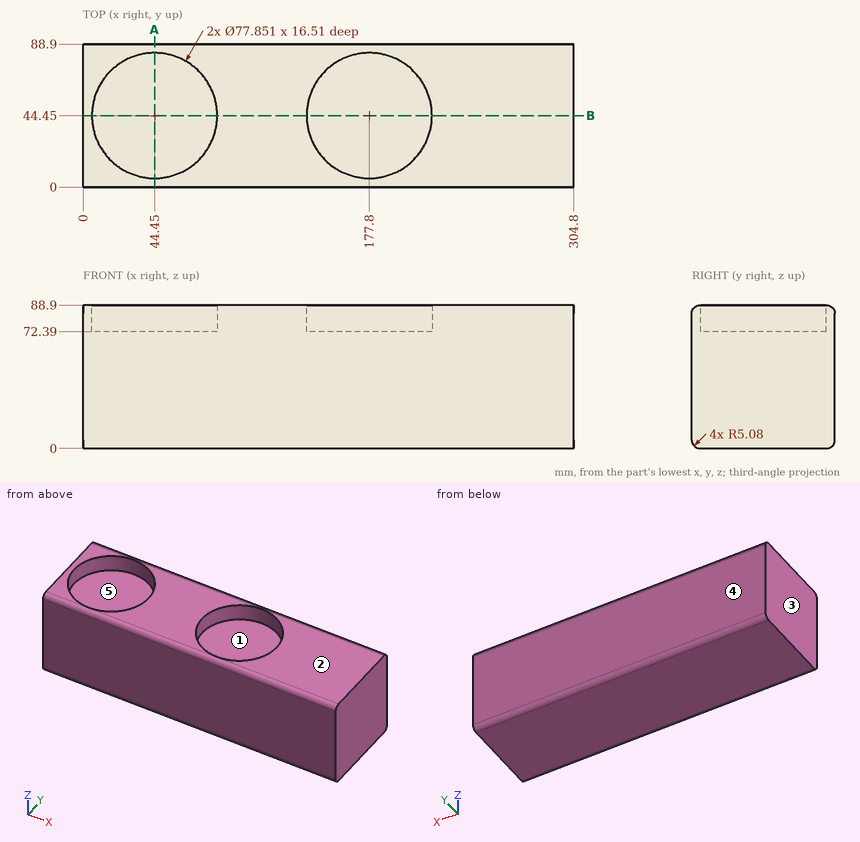
Here's the drawing with two shaded views (mm, measured from the low corner). I have some questions. A direction names the side the tool comes from. Round coordinates to 2 decimals unless told otherwise and drop trailing zeros. Write each loop counter-clockwise with the first axis right and the second up, starting at its lowest first coordinate (ties: lowest second). Pieces come first, ordered by that corner, then holes. Notation, with made-up numbers: M -18,14 L -12,14 A20 cw -12,22 Z; hole C -20,34.5 d9. An arc over 180 degrees is marked long. Use CSV: the item, a comma, the result in double quotes.
(1) I'm going to push flat-ended pins straight in: pin 1 (8 mm diameter, centred on x = 180, z = 49.5, fed in from -Y); pin 2 (1.5 mm diameter, centred on x = 210, y = 33, fed in from +Z). Where does each tip first touch, or does it pass through?
Check values:
pin 1,"y = 0"
pin 2,"z = 72.39"
(2) Imagine slicing it at A-A (x = 44.45). Write out the boundary of the cut face in (y, z).
Check values:
outline,"M 0,5.08 A5.08 ccw 5.08,0 L 83.82,0 A5.08 ccw 88.9,5.08 L 88.9,83.82 A5.08 ccw 83.82,88.9 L 83.38,88.9 L 83.38,72.39 L 5.52,72.39 L 5.52,88.9 L 5.08,88.9 A5.08 ccw 0,83.82 Z"
(3) We'd pull the mould along X, two halves only. Please class the marked faces 1, 2 and 3: +X half, -X half, draft (parallel to the pull), parting line (faces both ways), or undercut.
Check values:
face 1,"undercut"
face 2,"draft"
face 3,"-X half"
(4) I need wall thicknesses on line 1 along Y through (x, z) = (44.45, 77); line 2 along Z through (x, y) = (62, 77.5); line 3 along Y through (x, z) = (182, 72.5). Which ranges of each line are inside material? Lowest first, please.
Check values:
line 1,"0 to 5.52, 83.38 to 88.9"
line 2,"0 to 72.39"
line 3,"0 to 5.75, 83.15 to 88.9"
(5) Imagine slicing it at B-B (y = 44.45). Write out the boundary of the cut face in (x, z), plus the area to 3 significant figures.
Check values:
outline,"M 0,0 L 304.8,0 L 304.8,88.9 L 216.73,88.9 L 216.73,72.39 L 138.87,72.39 L 138.87,88.9 L 83.38,88.9 L 83.38,72.39 L 5.52,72.39 L 5.52,88.9 L 0,88.9 Z"
area,"24,500 mm^2"
(6) On a 3-axis mill with a long thin cutter (end or side, diameter ignored), from which of +Z, -Z, +X, -X, +Y, -Y can I reach the whole of each face in a straight line? I mean the marked faces 4 and 5. Say none if no direction works.
Check values:
face 4,"+Z, -Z, +X, -X, +Y"
face 5,"+Z"
